Geometry: see drawing. Coordinates: mm, zero at the bounding-box minimum. Give positions to 0.01 mm unless a question says otherwise; leave off trailing zeros. Write each loop counter-clockwise with the first axis right and the second up, starting at its lowest first coordinate (ties: lowest second). Pieces come first, ordered by that corner, then holes. Notation, with made-up numbers: (-20.5, -4) -> (17.5, -4) arc R26 cw to (17.5, 15) -> close; hole circle Ø5 at (75, -26). An arc over 180 degrees is marked (long way). Write item = value, one per line.
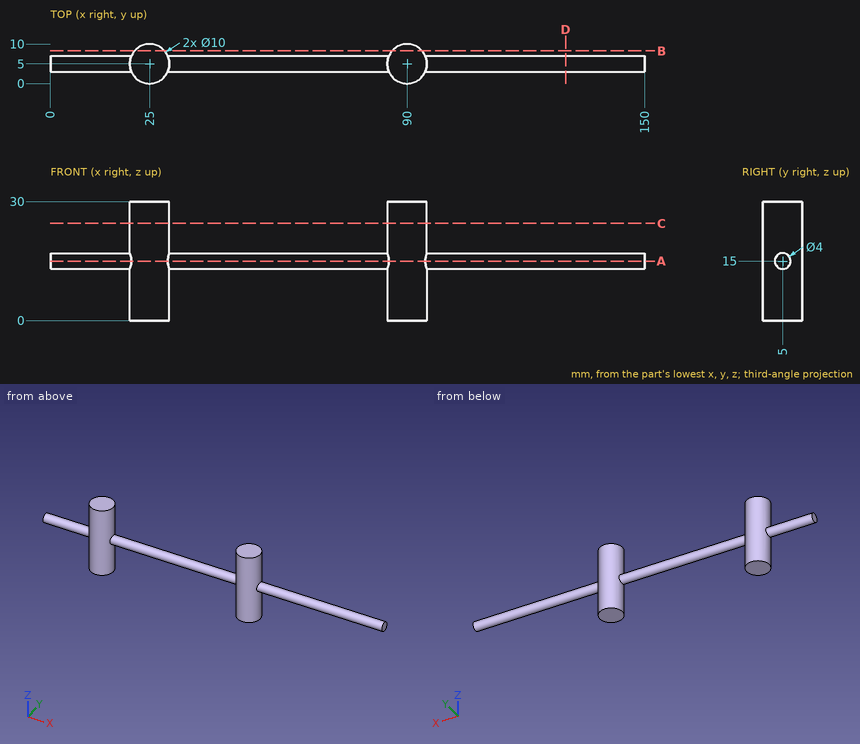
(1) Material intervals for line 1 (X direction, y = 3, z = 22); line 2 (X direction, y = 1, z = 13.5); line 3 (Y direction, x = 70, z = 16.5), sorted ascending.
Values follow:
line_1 = 20.42 to 29.58, 85.42 to 94.58
line_2 = 22 to 28, 87 to 93
line_3 = 3.68 to 6.32
(2) Section query A-A (z = 15). Return loops of the section in (x, y), plus the area to 3 significant figures.
Values follow:
outline = (0, 3) -> (20.42, 3) arc R5 ccw to (29.58, 3) -> (85.42, 3) arc R5 ccw to (94.58, 3) -> (150, 3) -> (150, 7) -> (94.58, 7) arc R5 ccw to (85.42, 7) -> (29.58, 7) arc R5 ccw to (20.42, 7) -> (0, 7) -> close
area = 679 mm2
(3) First-contact query: pin 1 (2 mm diameter, centred on x = 46.5, y = 7, fed in from +Z); pin 2 (2 mm diameter, centred on x = 103, y = 3, fed in from -Z); pin 3 (5 mm diameter, centred on x = 121, y = 3, fed in from +Z). Flat tips, straight axial feed; report the tip coordinate or a pass-through.
Values follow:
pin_1 = 16.73
pin_2 = 13.27
pin_3 = 17
(4) Section query D-D (x = 130). Return loops of the section in (y, z).
Values follow:
outline = circle Ø4 at (5, 15)
(5) Section query B-B (y = 8.25). Return loops of the section in (x, z).
Values follow:
outline = (21.2, 0) -> (28.8, 0) -> (28.8, 30) -> (21.2, 30) -> close; (86.2, 0) -> (93.8, 0) -> (93.8, 30) -> (86.2, 30) -> close
(6) Section query C-C (z = 24.5). Return loops of the section in (x, y).
Values follow:
outline = circle Ø10 at (25, 5); circle Ø10 at (90, 5)
